Model file for the job. Use its own axes, mm. Round coordinates to 2 decimals unless told otherwise and drop trailing zeros. Loops run counter-clockwise (first coordinate to the right, second up) from the corner with the lowest first, then second, coordinate; pieces in that order, holes last. Notation, with made-up numbers: (42, 18) -> (60, 18) arc R30 cw to (60, 52) -> close; hole circle Ø9 at (34.5, 88.25). An arc over 180 degrees is marked (long way). Use a Markdown table: item, result.
from build123d import *

# Parameters (mm, degrees)
CROQUIS1_R              = 11.73
SALIENTE_EXTRUIR1_DEPTH = 100
CROQUIS2_R              = 11.23
CORTAR_EXTRUIR1_DEPTH   = 102.366591143
REDONDEO1_R             = 0.5
REDONDEO4_R             = 0.5


with BuildPart() as part:
    # Croquis1 → Saliente-Extruir1 (new body)
    with BuildSketch(Plane(origin=(0, 0, 0), x_dir=(1, 0, 0), z_dir=(0, 1, 0))):
        with Locations(Location((0, 0, 0), (0, 0, 270))):
            Circle(CROQUIS1_R)
    extrude(amount=SALIENTE_EXTRUIR1_DEPTH)

    # Croquis2 → Cortar-Extruir1 (cut, through all)
    with BuildSketch(Plane(origin=(0, 100, 0), x_dir=(1, 0, 0), z_dir=(0, 1, 0))):
        with Locations(Location((0, 0, 0), (0, 0, 270))):
            Circle(CROQUIS2_R)
    extrude(amount=-CORTAR_EXTRUIR1_DEPTH, mode=Mode.SUBTRACT)

    # Redondeo1
    redondeo1_edges = [part.edges().sort_by_distance(p)[0] for p in [
        (0, 100, -11.73),
    ]]
    fillet(redondeo1_edges, radius=REDONDEO1_R - 0.0001)  # a hair under: the kernel refuses the full size

    # Redondeo4
    redondeo4_edges = [part.edges().sort_by_distance(p)[0] for p in [
        (0, 0, -11.73),
    ]]
    fillet(redondeo4_edges, radius=REDONDEO4_R - 0.0001)  # a hair under: the kernel refuses the full size


solid = part.part
Q1. Band-saw the part on C-C, the plane y = 56. Give the cut face in (x, z).
Results list:
| item | result |
|---|---|
| outline | circle Ø23.46 at (0, 0); hole circle Ø22.46 at (0, 0) |
Q2. Drill centre lines: L1, parallel to X at y = 26.5, z = 0; L2, parallel to X at y = 27.5, z = 6. Where is each one in solid material? Low to high. Write a range as from..to.
Results list:
| item | result |
|---|---|
| L1 | x = -11.73..-11.23, 11.23..11.73 |
| L2 | x = -10.08..-9.49, 9.49..10.08 |
Q3. Pull direction Z, two halves, no side cores. Call faces 1 (the face through (-10.41, 49.31, 5.41)), 2 (the face through (11.134, 50.7, -1.462)): released by +Z, released by -Z, zero draft, split by the parting line, or undercut.
Results list:
| item | result |
|---|---|
| face 1 | split by the parting line |
| face 2 | undercut |
Q4. Flat gauge pins, fed straight in: pin 1 (4 mm diameter, centred on x = -3, y = 62.5, fed in from +Z); pin 2 (6 mm diameter, centred on y = 34, z = -1, fed in from -X); pin 3 (8 mm diameter, centred on y = 21, z = -7, fed in from +X). Where does each tip first touch, or does it go through?
Results list:
| item | result |
|---|---|
| pin 1 | stops at z = 11.69 |
| pin 2 | stops at x = -11.73 |
| pin 3 | stops at x = 11.34 |
